```python
from build123d import *

# Parameters (mm, degrees)
F1_DEPTH = 250
F2_DEPTH = 232


with BuildPart() as f1:
    # F0 (on Front) → F1 (new body, symmetric)
    with BuildSketch(Plane.XZ):
        Polygon((-198.168553, 183.939874), (-216.168553, 183.939874), (-216.168553, -316.060126), (283.831447, -316.060126), (283.831447, -298.060126), (-198.168553, -298.060126), align=None)
        Polygon((283.831447, -298.060126), (-198.168553, 183.939874), (-198.168553, -298.060126), align=None)
    extrude(amount=F1_DEPTH, both=True)

    # F0 (on Front) → F2 (cut, symmetric)
    with BuildSketch(Plane.XZ):
        Polygon((283.831447, 183.939874), (-198.168553, 183.939874), (283.831447, -298.060126), align=None)
        Polygon((283.831447, -298.060126), (-198.168553, 183.939874), (-198.168553, -298.060126), align=None)
    extrude(amount=F2_DEPTH, both=True, mode=Mode.SUBTRACT)


solid = f1.part
```
Here's how the part is built. I have some questions about the finished solid (model axes, mm). A direction names the side the tool comes from. Give positions to 0.01 mm unless a question says otherwise; leave off trailing zeros. Write each loop counter-clockwise with the first axis right and the second up, starting at its lowest first coordinate (ties: lowest second). Pieces come first, ordered by that corner, then holes. Notation, with made-up numbers: (-11.5, 31) -> (8.5, 31) arc R18 ccw to (8.5, 50) -> close; hole circle Ø2 at (58, 42.5). An arc over 180 degrees is marked (long way). Use one line per item in the form item = value.
1) If I drill on L1, parallel to Y at x = -94.5, z = -270; L2, parallel to X at y = 140.5, z = 122; L3, parallel to Z at x = -180, y = -4, over which ranges is the centre line in solid material (lowest first)? Write a range as [from, to].
Verdict:
L1 = [-250, -232], [232, 250]
L2 = [-216.17, -198.17]
L3 = [-316.06, -298.06]
2) On a 3-axis mill with a long thin cutter (end or side, diameter ignored), from which of +Z, -Z, +X, -X, +Y, -Y can I reach the whole of each face in a straight line? I mean faces 5 (the face through (46.205, -241.126, -60.434)), 6 (the face through (-198.169, -3, -54)). Say none if no direction works.
Verdict:
face_5 = +Z, +X, +Y, -Y
face_6 = +Z, +X
3) Suppose I cut it at A-A (z = -17.5). Please give me the cut outline in (x, y), and give its area (3 significant figures).
Verdict:
outline = (-216.17, -250) -> (3.27, -250) -> (3.27, -232) -> (-198.17, -232) -> (-198.17, 232) -> (3.27, 232) -> (3.27, 250) -> (-216.17, 250) -> close
area = 16,300 mm2
4) Suppose I cut it at C-C (y = 151). Please give me the cut outline in (x, z), and give its area (3 significant figures).
Verdict:
outline = (-216.17, -316.06) -> (283.83, -316.06) -> (283.83, -298.06) -> (-198.17, -298.06) -> (-198.17, 183.94) -> (-216.17, 183.94) -> close
area = 17,700 mm2
5) Suppose I cut it at B-B (x = -183.5). Please give me the cut outline in (y, z), and give its area (3 significant figures).
Verdict:
outline = (-250, -316.06) -> (250, -316.06) -> (250, 169.27) -> (232, 169.27) -> (232, -298.06) -> (-232, -298.06) -> (-232, 169.27) -> (-250, 169.27) -> close
area = 25,800 mm2
6) I'm going to push flat-ended pins straight in: pin 1 (5 mm diameter, centred on y = 187.5, z = 22, fed in from +X); pin 2 (3 mm diameter, centred on x = -107, y = 197, fed in from +Z). Where does each tip first touch, or does it pass through?
Verdict:
pin_1 = -198.17
pin_2 = -298.06
7) We'd pull the mould along Y, two halves only. Please class faces 1 (the face through (-25, -250, -118)), 2 (the face through (-68, 232, -161)), 3 (the face through (-68, -232, -161)), 4 (the face through (-216.169, -4, -63)): +Y half, -Y half, draft (parallel to the pull), parting line (faces both ways), or undercut.
Verdict:
face_1 = -Y half
face_2 = undercut
face_3 = undercut
face_4 = draft
